For this review, take the finished solid that the model builds, in its own axes (mm). Coordinates: 2 decimals unless noted, no trailing zeros. Order: outer loops, then holes, each group sorted by start corner. A loop starts at its lowest first (then second) coordinate and runs counter-clockwise, first axis right, second up. Notation, with made-up numbers: (27.5, 26) - (50.5, 26) arc R27 cw to (50.5, 42) - close; hole circle Ø7 at (78.5, -1). An arc over 180 degrees is marked (long way). One line per item, written item: value. Start each with the question number.
(1) To check wall thickness, follow line 1 along Z through (x, y) = (-66, -2.25); line 2 along X through (y, z) = (-1.35, 0). State the ranges of each line that lie inside material, in increasing order.
(2) Consider section B-B on y = -1.65. Write out the cut boundary in (x, z).
(3) Consider section C-C on x = 6. Write out the cut boundary in (y, z) (3 decimals), then the cut area to 3 significant figures.
(4) Consider section A-A on z = 4.5. Write out the cut boundary in (x, y) (3 decimals).
```python
from build123d import *

# Parameters (mm, degrees)
F0_W     = 304.8
F0_H     = 203.2
F1_DEPTH = 3.175
F2_W     = 177.8
F2_H     = 63.5
F3_DEPTH = 12.7


with BuildPart() as f1:
    # F0 (on Front) → F1 (new body)
    with BuildSketch(Plane.XZ):
        Rectangle(F0_W, F0_H)
    extrude(amount=F1_DEPTH)

    # F2 (on face) → F3 (cut, symmetric)
    with BuildSketch(Plane(origin=(0, 0, 0), x_dir=(-1, 0, 0), z_dir=(0, 1, 0))):
        Rectangle(F2_W, F2_H)
    extrude(amount=F3_DEPTH, both=True, mode=Mode.SUBTRACT)


solid = f1.part
```
Geometry check:
1. line 1: z = -101.6 to -31.75, 31.75 to 101.6
1. line 2: x = -152.4 to -88.9, 88.9 to 152.4
2. outline: (-152.4, -101.6) - (152.4, -101.6) - (152.4, 101.6) - (-152.4, 101.6) - close; hole (-88.9, -31.75) - (88.9, -31.75) - (88.9, 31.75) - (-88.9, 31.75) - close
3. outline: (-3.175, -101.6) - (0, -101.6) - (0, -31.75) - (-3.175, -31.75) - close; (-3.175, 31.75) - (0, 31.75) - (0, 101.6) - (-3.175, 101.6) - close
3. area: 444 mm^2
4. outline: (-152.4, -3.175) - (-88.9, -3.175) - (-88.9, 0) - (-152.4, 0) - close; (88.9, -3.175) - (152.4, -3.175) - (152.4, 0) - (88.9, 0) - close
